from build123d import *

# Parameters (mm, degrees)
F0_R      = 2.5
F0_W      = 1.9671103259
F0_H      = 32.8726123017
F1_DEPTH  = 23
F0_W_2    = 10
F0_H_2    = 2
F2_DEPTH  = 2
F3_DEPTH  = 21
F5_DEPTH  = 2
F3_FACE_W = 2
F3_FACE_H = 47.3760884154
F2_FACE_W = 10
F2_FACE_H = 2
F5_FACE_W = 10
F5_FACE_H = 2
F9_W      = 10
F9_H      = 22
F9_R      = 1.5
F10_DEPTH = 2


with BuildPart() as f1:
    # F0 (on Front) → F1 (new body, symmetric)
    with BuildSketch(Plane.XZ):
        with BuildLine():
            add(Edge.make_bspline(
                [(-41.9375598431, 64.1377046704), (-51.2842722237, 47.7368719876), (-55.3985677235, 50.4242394975), (-57.4354853918, 38.2308801777)],
                knots=[0, 0, 0, 0, 30.1885616022, 30.1885616022, 30.1885616022, 30.1885616022], degree=3))
            Line((-57.4354853918, 38.2308801777), (-57.4354853918, 5.358267876))
            Line((-57.4354853918, 5.358267876), (-31.1536770314, -34.0594984591))
            add(Edge.make_bspline(
                [(-21.304015945, 20.5783754124), (-34.3524827141, 3.69984575), (-31.5767975227, -1.8766191306), (-31.1536770314, -34.0594984591)],
                knots=[0, 0, 0, 0, 56.0586211891, 56.0586211891, 56.0586211891, 56.0586211891], degree=3))
            Line((-21.304015945, 20.5783754124), (-19.717078656, 30.4542761296))
            Line((-19.717078656, 30.4542761296), (-25.1840222627, 40.1536934078))
            add(Edge.make_bspline(
                [(-41.9375598431, 64.1377046704), (-34.8834395409, 55.6727573276), (-36.6469696164, 50.3821708262), (-25.1840222627, 40.1536934078)],
                knots=[0, 0, 0, 0, 29.2560048145, 29.2560048145, 29.2560048145, 29.2560048145], degree=3))
        make_face()
        with Locations((-36.313764751, 30.7701863348)):
            Circle(F0_R, mode=Mode.SUBTRACT)
        with Locations((-58.4190405548, 21.7945740269)):
            Rectangle(F0_W, F0_H)
    extrude(amount=F1_DEPTH, both=True)

    # F0 (on Front) → F3 (cut, symmetric)
    with BuildSketch(Plane.XZ):
        with BuildLine():
            add(Edge.make_bspline(
                [(-41.9375598431, 64.1377046704), (-51.2842722237, 47.7368719876), (-55.3985677235, 50.4242394975), (-57.4354853918, 38.2308801777)],
                knots=[0, 0, 0, 0, 30.1885616022, 30.1885616022, 30.1885616022, 30.1885616022], degree=3))
            Line((-57.4354853918, 38.2308801777), (-57.4354853918, 5.358267876))
            Line((-57.4354853918, 5.358267876), (-31.1536770314, -34.0594984591))
            add(Edge.make_bspline(
                [(-21.304015945, 20.5783754124), (-34.3524827141, 3.69984575), (-31.5767975227, -1.8766191306), (-31.1536770314, -34.0594984591)],
                knots=[0, 0, 0, 0, 56.0586211891, 56.0586211891, 56.0586211891, 56.0586211891], degree=3))
            Line((-21.304015945, 20.5783754124), (-19.717078656, 30.4542761296))
            Line((-19.717078656, 30.4542761296), (-25.1840222627, 40.1536934078))
            add(Edge.make_bspline(
                [(-41.9375598431, 64.1377046704), (-34.8834395409, 55.6727573276), (-36.6469696164, 50.3821708262), (-25.1840222627, 40.1536934078)],
                knots=[0, 0, 0, 0, 29.2560048145, 29.2560048145, 29.2560048145, 29.2560048145], degree=3))
        make_face()
        with Locations((-36.313764751, 30.7701863348)):
            Circle(F0_R, mode=Mode.SUBTRACT)
    extrude(amount=F3_DEPTH, both=True, mode=Mode.SUBTRACT)



with BuildPart() as f2:
    # F0 (on Front) → F2 (new body)
    with BuildSketch(Plane.XZ):
        with Locations((-32.0685834799, -93.5112637015)):
            Rectangle(F0_W_2, F0_H_2)
    extrude(amount=F2_DEPTH)


with BuildPart() as f2_1:
    # F4: moved
    add(f2.part.moved(Location((0, -10, 0))))


with BuildPart() as f5:
    # F0 (on Front) → F5 (new body)
    with BuildSketch(Plane.XZ):
        with Locations((-32.0685834799, -93.5112637015)):
            Rectangle(F0_W_2, F0_H_2)
    extrude(amount=-F5_DEPTH)


with BuildPart() as f5_1:
    # F6: moved
    add(f5.part.moved(Location((0, 10, 0))))


with BuildPart() as f1_1:
    add(f1.part)

    add(f2_1.part)  # F7 merges F2
    # F3_face (on face) → F7 section 0
    with BuildSketch(Plane(origin=(-44.2945812116, -22, -14.3506152915), x_dir=(0, -1, 0), z_dir=(-0.8320181689, 0, -0.5547483813))):
        Rectangle(F3_FACE_W, F3_FACE_H)
    # F2_face (on face) → F7 section 1
    with BuildSketch(Plane(origin=(-32.0685834799, -11, -92.5112637015), x_dir=(1, 0, 0), z_dir=(0, 0, 1))):
        Rectangle(F2_FACE_W, F2_FACE_H)
    loft()


    add(f5_1.part)  # F8 merges F5
    # F3_face (on face) → F8 section 0
    with BuildSketch(Plane(origin=(-44.2945812116, -22, -14.3506152915), x_dir=(0, -1, 0), z_dir=(-0.8320181689, 0, -0.5547483813))):
        with Locations((-44, 0)):
            Rectangle(F3_FACE_W, F3_FACE_H)
    # F5_face (on face) → F8 section 1
    with BuildSketch(Plane(origin=(-32.0685834799, 11, -92.5112637015), x_dir=(1, 0, 0), z_dir=(0, 0, 1))):
        Rectangle(F5_FACE_W, F5_FACE_H)
    loft()

    # F9 (on face) → F10 (join)
    with BuildSketch(Plane(origin=(0, 0, -94.5112637015), x_dir=(1, 0, 0), z_dir=(0, 0, -1))):
        with Locations((-32.0685834799, -1)):
            Rectangle(F9_W, F9_H)
        with Locations((-32.0685834799, -5)):
            Circle(F9_R, mode=Mode.SUBTRACT)
        with Locations((-32.0685834799, 5)):
            Circle(F9_R, mode=Mode.SUBTRACT)
    extrude(amount=-F10_DEPTH)


solid = f1_1.part
CAD build for the part. Positions are in the model's coordinates, mm. A direction names the side the tool comes from. Coordinates: 2 decimals unless noted, no trailing zeros. Loops run counter-clockwise (first coordinate to the right, second up) from the corner with the lowest first, then second, coordinate; pieces in that order, holes last. Notation, with made-up numbers: (24.5, 24) - (61.5, 24) arc R33 cw to (61.5, 63) - close; hole circle Ø10 at (23, 69). An arc over 180 degrees is marked (long way). Use one line per item in the form item = value. Start each with the question number.
1) Drill centre lines: L1, parallel to Y at x = -34, z = -11.5; L2, parallel to X at y = -5, z = -93.15; L3, parallel to Y at x = -30, z = -58.5. Where is each one in solid material? Low to high. Write a range as from..to.
2) Band-saw the part on A-A (y = 5). Give the cut face in (x, z).
3) Flat gauge pins, fed straight in: pin 1 (16.5 mm diameter, centred on y = 2, z = 29.5, fed in from +X); pin 2 (1 mm diameter, centred on x = -29.5, z = -93.5, fed in from +Y); pin 3 (2 mm diameter, centred on y = -1, z = -94, fed in from +X). Where does each tip first touch, or does it go through?
4) Tool access for faces 1 (the face through (-57.435, 0, 22)), 2 (the face through (-33.567, -5.066, -93.525)), 3 (the face through (-39, 21, 27)): list every direction of +Z, -Z, +X, -X, +Y, -Y with a clear straight run to the whole face (end or side of a thin tool).
5) Two-plate mould, pull along Y, no slides. Class faces 4 (the face through (-40, -23, 27)), 5 (the face through (-32, 0, -92.511)), 6 (the face through (-33.567, 4.934, -93.525)), 7 (the face through (-59.403, 0, 22)): +Y half, -Y half, draft (parallel to the pull), parting line (faces both ways), or undercut.
Check values:
q1.L1 = -23..-21, 21..23
q1.L2 = -37.07..-33.57, -30.57..-27.07
q1.L3 = -18.27..-16.27, 16.27..18.27
q2.outline = (-59.4, 5.36) - (-57.44, 5.36) - (-57.44, 38.23) - (-59.4, 38.23) - close; (-37.07, -94.51) - (-33.57, -94.51) - (-33.57, -92.51) - (-37.07, -92.51) - close; (-30.57, -94.51) - (-27.07, -94.51) - (-27.07, -92.51) - (-30.57, -92.51) - close
q3.pin_1 = -57.44
q3.pin_2 = 12
q3.pin_3 = -27.07
q4.face_1 = +Z, -Z, +X
q4.face_2 = +Z, -Z
q4.face_3 = +Z, +X
q5.face_4 = -Y half
q5.face_5 = undercut
q5.face_6 = undercut
q5.face_7 = draft
